from build123d import *

# Parameters (mm, degrees)
BOSS_EXTRUDE1_DEPTH = 19.05
SKETCH8_R           = 6.35
CUT_EXTRUDE3_DEPTH  = 1152.453768969
CUT_EXTRUDE4_DEPTH  = 1152.453768969
SKETCH10_R          = 6.35
CUT_EXTRUDE5_DEPTH  = 1152.453768969


with BuildPart() as part:
    # Sketch1 → Boss-Extrude1 (new body)
    with BuildSketch(Plane.XY):
        Polygon((-10.620091868, 228.043424569), (1088.227150324, 343.536923634), (1098.847242192, 242.493499064), (1098.847242192, 0), (0, 0), (0, 127), align=None)
    extrude(amount=BOSS_EXTRUDE1_DEPTH)

    # Sketch8 → Cut-Extrude3 (cut, through all)
    with BuildSketch(Plane.XY.offset(19.05)):
        with Locations((86.197214357, 157.1625)):
            Circle(SKETCH8_R)
        with BuildLine():
            Line((442.415992192, 161.13125), (536.078492192, 161.13125))
            ThreePointArc((536.078492192, 161.13125), (540.047242192, 157.1625), (536.078492192, 153.19375))
            Line((536.078492192, 153.19375), (442.415992192, 153.19375))
            ThreePointArc((442.415992192, 153.19375), (438.447242192, 157.1625), (442.415992192, 161.13125))
        make_face()
    extrude(amount=-CUT_EXTRUDE3_DEPTH, mode=Mode.SUBTRACT)

    # Sketch9 → Cut-Extrude4 (cut, through all)
    with BuildSketch(Plane.XY.offset(19.05)):
        with BuildLine():
            ThreePointArc((1035.904292432, 85.7708681), (1030.742924963, 184.255626282), (1015.315371576, 281.661364844))
            ThreePointArc((1015.315371576, 281.661364844), (1012.491067888, 283.495489105), (1010.656943627, 280.671185417))
            ThreePointArc((1010.656943627, 280.671185417), (1026.006514436, 183.757809476), (1031.141792432, 85.7708681))
            ThreePointArc((1031.141792432, 85.7708681), (1033.523042432, 83.3896181), (1035.904292432, 85.7708681))
        make_face()
    extrude(amount=-CUT_EXTRUDE4_DEPTH, mode=Mode.SUBTRACT)

    # Sketch10 → Cut-Extrude5 (cut, through all)
    with BuildSketch(Plane.XY.offset(19.05)):
        with Locations((946.447242192, 88.9)):
            Circle(SKETCH10_R)
    extrude(amount=-CUT_EXTRUDE5_DEPTH, mode=Mode.SUBTRACT)


solid = part.part
Read the model definition and answer for the solid it produces. Units are mm, in the model's axes. A direction names the side the tool comes from. Round coordinates to 2 decimals unless told otherwise and drop trailing zeros. Order: outer loops, then holes, each group sorted by start corner. A loop starts at its lowest first (then second) coordinate and runs counter-clockwise, first axis right, second up. Notation, with made-up numbers: (84, -14) - (116, -14) arc R31 ccw to (116, 23) - close; hole circle Ø3 at (-17, -33.5). An arc over 180 degrees is marked (long way). Use one line per item in the form item = value. Start each with the question number.
(1) The part is cut by section C-C (x = 989.5). Give the vertices of the cut face in (y, z), then the cut area to 3 significant figures.
(2) The part is cut by section B-B (x = 642). Give the vertices of the cut face in (y, z), then the cut area to 3 significant figures.
(3) Flat-ended cylindrical pins translate along their axes: pin 1 Ø1.5 at (y, z) = (309, 7) entering from +X; pin 2 Ø2 at (y, z) = (56.5, 5) entering from -X; pin 3 Ø9.5 at (x, z) = (485, 8) entering from +Y. Find the tip coordinate at first contact, or state that the pin passes through.
(4) Determine the mould class of faces 1 (the face through (531.11, 284.98, 9.39)), 2 (the face through (1093.463, 293.723, 9.392)), 3 (the face through (1025.862, 185.125, 9.658)) for opening direction X: +X half, -X half, draft (parallel to the pull), parting line (faces both ways), or undercut.
(5) Find the intervals of material crossed by line 1 along Y through (x, z) = (125, 12.5); line 2 along X through (y, z) = (106, 2.25); line 3 along X through (y, z) = (226, 10.75), in increasing order. Write a range as from..to.
(6) The part is cut by section A-A (z = 6). Give the vertices of the cut face in (x, y).
(7) For faces 4 (the face through (489, 161.131, 10)), 5 (the face through (0, 63, 9)), 6 (the face through (552, 136, 0)), determine the directions among +Z, -Z, +X, -X, +Y, -Y from which every point of the face is accessible in a straight line to the end or side of a thin tool.
Checked values:
q1.outline = (0, 0) - (333.16, 0) - (333.16, 19.05) - (0, 19.05) - close
q1.area = 6,350 mm^2
q2.outline = (0, 0) - (296.64, 0) - (296.64, 19.05) - (0, 19.05) - close
q2.area = 5,650 mm^2
q3.pin_1 = 1091.94
q3.pin_2 = 0
q3.pin_3 = 280.63
q4.face_1 = -X half
q4.face_2 = +X half
q4.face_3 = undercut
q5.line_1 = 0..242.3
q5.line_2 = 0..1030.92, 1035.69..1098.85
q5.line_3 = -10.41..1020.59, 1025.41..1098.85
q6.outline = (-10.62, 228.04) - (0, 127) - (0, 0) - (1098.85, 0) - (1098.85, 242.49) - (1088.23, 343.54) - close; hole circle Ø12.7 at (86.2, 157.16); hole (442.42, 153.19) - (536.08, 153.19) arc R3.97 ccw to (536.08, 161.13) - (442.42, 161.13) arc R3.97 ccw to start; hole circle Ø12.7 at (946.45, 88.9); hole (1010.66, 280.67) arc R937.42 cw to (1031.14, 85.77) arc R2.38 ccw to (1035.9, 85.77) arc R942.18 ccw to (1015.32, 281.66) arc R2.38 ccw to start
q7.face_4 = +Z, -Z
q7.face_5 = +Z, -Z, -X, -Y
q7.face_6 = -Z, +X, -X, +Y, -Y
